Input: part model. Units: mm. Frame: model coordinates. A direction names the side the tool comes from. Round coordinates to 2 decimals unless told otherwise and drop trailing zeros. Loops run counter-clockwise (first coordinate to the right, second up) from the corner with the lowest first, then second, coordinate; pieces in that order, holes last. Notation, with made-up numbers: (-30.75, 17) - (9.25, 17) arc R31 cw to (9.25, 49) - close; hole circle Ø3 at (-32.5, 16.25). An arc over 180 degrees is marked (long way). Write each question's results on one line, items separated by ' | '.
from build123d import *

# Parameters (mm, degrees)
BOSS_EXTRUDE1_DEPTH = 7.5
CUT_EXTRUDE1_DEPTH  = 39.405728739
BOSS_EXTRUDE3_DEPTH = 2.375
FILLET1_R           = 1
FILLET2_R           = 1
FILLET3_R           = 1
FILLET4_R           = 1
CHAMFER1_SIZE       = 1
CHAMFER2_SIZE       = 1


with BuildPart() as part:
    # Sketch1 → Boss-Extrude1 (new, symmetric)
    with BuildSketch(Plane.XY):
        with BuildLine():
            Line((-25, 0), (-15, 0))
            ThreePointArc((-15, 0), (0, 15), (15, 0))
            Line((15, 0), (25, 0))
            ThreePointArc((25, 0), (0, 25), (-25, 0))
        make_face()
    extrude(amount=BOSS_EXTRUDE1_DEPTH, both=True)

    # Sketch2 → Cut-Extrude1 (cut, through all)
    with BuildSketch(Plane.XY.offset(7.5)):
        Polygon((-22.625, 5.25), (-17.375, 5.25), (-18.425, 0), (-21.575, 0), align=None)
    cut_extrude1 = extrude(amount=-CUT_EXTRUDE1_DEPTH, mode=Mode.SUBTRACT)

    # Mirror1: Cut-Extrude1 across plane
    add(cut_extrude1.mirror(Plane(origin=(0, 0, 0), x_dir=(0, 0, 1), z_dir=(1, 0, 0))), mode=Mode.SUBTRACT)

    # Sketch3 → Boss-Extrude3 (add, symmetric)
    with BuildSketch(Plane.XY):
        with BuildLine():
            Line((12.475, 8.329128106), (12.475, -5.7))
            Line((12.475, -5.7), (11.475, -5.7))
            Line((11.475, -5.7), (11.475, -10.7))
            Line((11.475, -10.7), (16.425, -10.7))
            Line((16.425, -10.7), (16.425, -7.85))
            Line((16.425, -7.85), (15.475, -5.95))
            Line((15.475, -5.95), (15.475, 0))
            Line((15.475, 0), (15, 0))
            ThreePointArc((15, 0), (14.35487722, 4.351723796), (12.475, 8.329128106))
        make_face()
    boss_extrude3 = extrude(amount=BOSS_EXTRUDE3_DEPTH, both=True)

    # Mirror11: Boss-Extrude3 across plane
    add(boss_extrude3.mirror(Plane(origin=(0, 0, 0), x_dir=(0, 0, 1), z_dir=(1, 0, 0))))

    # Fillet1
    fillet1_edges = [part.edges().sort_by_distance(p)[0] for p in [
        (16.425, -10.7, 0),
    ]]
    fillet(fillet1_edges, radius=FILLET1_R)

    # Fillet2
    fillet2_edges = [part.edges().sort_by_distance(p)[0] for p in [
        (-16.425, -10.7, 0),
    ]]
    fillet(fillet2_edges, radius=FILLET2_R)

    # Fillet3
    fillet3_edges = [part.edges().sort_by_distance(p)[0] for p in [
        (-12.475, -5.7, 0),
    ]]
    fillet(fillet3_edges, radius=FILLET3_R - 0.0001)  # a hair under: the kernel refuses the full size

    # Fillet4
    fillet4_edges = [part.edges().sort_by_distance(p)[0] for p in [
        (12.475, -5.7, 0),
    ]]
    fillet(fillet4_edges, radius=FILLET4_R - 0.0001)  # a hair under: the kernel refuses the full size

    # Chamfer1
    chamfer1_edges = [part.edges().sort_by_distance(p)[0] for p in [
        (-20, 5.25, 7.5),
        (-22.1, 2.625, 7.5),
        (-17.9, 2.625, 7.5),
    ]]
    chamfer(chamfer1_edges, length=CHAMFER1_SIZE)

    # Chamfer2
    chamfer2_edges = [part.edges().sort_by_distance(p)[0] for p in [
        (22.1, 2.625, 7.5),
        (17.9, 2.625, 7.5),
        (20, 5.25, 7.5),
    ]]
    chamfer(chamfer2_edges, length=CHAMFER2_SIZE)


solid = part.part
1. Mould query, pull axis Y, two halves, no side actions, for faces 1 (the cylindrical face through (-16.124, -10.415, 0.033)), 2 (the flat face through (12.475, 2, 0)), 3 (the flat face through (11.475, -8, 0)). Classes: pulls with the +Y half, pulls with the -Y half, needs draft (parallel to the pull), parting line crosses it, or undercut.
Answer:
face 1: pulls with the -Y half | face 2: undercut | face 3: needs draft
2. Contact query for flat-ended pins moving along their axis: pin 1 (2 mm diameter, centred on y = 13.5, z = 1, fed in from -X); pin 2 (2.5 mm diameter, centred on x = 24, z = -1, fed in from -Y); pin 3 (5 mm diameter, centred on y = -3, z = -0.5, fed in from +X) (3 decimals). Output: stop coordinate, or through.
Answer:
pin 1: x = -21.65 | pin 2: y = 0 | pin 3: x = 15.475
3. Section query C-C, the plane x = 0. Output: boundary loops of the cut face in (y, z), plus the area to 3 significant figures.
Answer:
outline: (15, -7.5) - (25, -7.5) - (25, 7.5) - (15, 7.5) - close | area: 150 mm^2
4. Set-up query: faces 4 (the flat face through (16.425, -9, 0)), 5 (the flat face through (14, -3, 2.375)), 6 (the flat face through (-22.093, 2.588, -0.402)), 7 (the flat face through (-17.29, 3.17, 6.99)), 8 (the flat face through (14, -3, -2.375)). Return all of +Z, -Z, +X, -X, +Y, -Y with unobstructed straight access to the full face (end or side cutting, diameter ignored); none if empty.
Answer:
face 4: +Z, -Z, +X, -Y | face 5: +Z, -Y | face 6: +Z, -Z | face 7: +Z | face 8: -Z, -Y
5. Section query D-D, the plane z = -5.75. Output: boundary loops of the cut face in (x, y) (3 decimals), plus the area to 3 significant figures.
Answer:
outline: (-25, 0) - (-21.575, 0) - (-22.625, 5.25) - (-17.375, 5.25) - (-18.425, 0) - (-15, 0) arc R15 cw to (15, 0) - (18.425, 0) - (17.375, 5.25) - (22.625, 5.25) - (21.575, 0) - (25, 0) arc R25 ccw to start | area: 584 mm^2
6. Section query B-B, the plane y = 4.5. Output: boundary loops of the cut face in (x, z) (3 decimals).
Answer:
outline: (-24.592, -7.5) - (-22.475, -7.5) - (-22.475, 6.5) - (-23.495, 7.5) - (-24.592, 7.5) - close; (-17.525, -7.5) - (-14.309, -7.5) - (-14.309, -2.375) - (-12.475, -2.375) - (-12.475, 2.375) - (-14.309, 2.375) - (-14.309, 7.5) - (-16.505, 7.5) - (-17.525, 6.5) - close; (12.475, -2.375) - (14.309, -2.375) - (14.309, -7.5) - (17.525, -7.5) - (17.525, 6.5) - (16.505, 7.5) - (14.309, 7.5) - (14.309, 2.375) - (12.475, 2.375) - close; (22.475, -7.5) - (24.592, -7.5) - (24.592, 7.5) - (23.495, 7.5) - (22.475, 6.5) - close
7. Line query: line 1 (X direction, y = 2, z = 5.5) (3 decimals); line 2 (X direction, y = 3, z = 2.5) (3 decimals); line 3 (X direction, y = -4.5, z = -0.25) (3 decimals). Output: solid intervals per line, ascending. Write a range as [from, to].
Answer:
line 1: [-24.92, -21.975], [-18.025, -14.866], [14.866, 18.025], [21.975, 24.92] | line 2: [-24.819, -22.175], [-17.825, -14.697], [14.697, 17.825], [22.175, 24.819] | line 3: [-15.475, -12.475], [12.475, 15.475]
